Here's how the part is built. I have some questions about the finished solid (model axes, mm). A direction names the side the tool comes from. Round coordinates to 2 decimals unless told otherwise and drop trailing zeros. Order: outer loops, then holes, each group sorted by start corner. A loop starts at its lowest first (then second) coordinate and runs counter-clockwise, first axis right, second up. Notation, with made-up numbers: (1, -9.5) -> (47, -9.5) arc R19 cw to (47, 7.5) -> close; hole circle Ø5 at (-5, 15.5). An arc over 180 degrees is marked (long way). Use a Markdown table: item, result. Add a question column.
from build123d import *

# Parameters (mm, degrees)
F0_W     = 38.1
F0_H     = 31.75
F1_DEPTH = 25.4
F2_W     = 12.7
F2_H     = 19.3866453245
F3_DEPTH = 25.4
F5_DEPTH = 25.4
F7_DEPTH = 25.4


with BuildPart() as f1:
    # F0 (on Right) → F1 (new body)
    with BuildSketch(Plane.YZ):
        with Locations((19.05, 15.875)):
            Rectangle(F0_W, F0_H)
    extrude(amount=F1_DEPTH)

    # F2 (on face) → F3 (cut)
    with BuildSketch(Plane.YZ.offset(25.4)):
        with Locations((6.35, 22.0566773377)):
            Rectangle(F2_W, F2_H)
    extrude(amount=-F3_DEPTH, mode=Mode.SUBTRACT)

    # F4 (on face) → F5 (cut)
    with BuildSketch(Plane(origin=(0, 38.1, 0), x_dir=(-1, 0, 0), z_dir=(0, 1, 0))):
        Polygon((-25.4, 10.1520223543), (-12.7, 31.75), (-25.4, 31.75), align=None)
    extrude(amount=-F5_DEPTH, mode=Mode.SUBTRACT)

    # F6 (on face) → F7 (cut)
    with BuildSketch(Plane.XY.offset(12.3633546755)):
        Polygon((25.4, 0), (25.4, 12.7), (12.7, 0), align=None)
    extrude(amount=-F7_DEPTH, mode=Mode.SUBTRACT)


solid = f1.part
(1) On a 3-axis mill with a long thin cutter (end or side, diameter ignored), from which of +Z, -Z, +X, -X, +Y, -Y can I reach the whole of each face in a straight line? I mean faces 1 (the flat face through (10, 12.7, 22)), 2 (the flat face through (25, 12.7, 12)), 3 (the flat face through (25.4, 25, 5)). Say none if no direction works.
(2) I want a section at C-C on z = 3.5. List the corners of the cut face in (x, y) for me.
(3) I want a section at A-A on y = 32.5. List the corners of the cut face in (x, z) for me.
(4) I want a section at D-D on y = 10. List the corners of the cut face in (x, z) for me, and give its area (3 significant figures).
(5) Please list where these lines run through material, in increasing order: probe 1 along Z at (x, y) = (14.5, 7); probe 2 along Y at (x, z) = (12, 17); probe 3 along Z at (x, y) = (16.75, 21). Write a range as from..to.
(6) I want a section at B-B on x = 9. List the corners of the cut face in (y, z) for me, and give its area (3 significant figures).
(7) I'm going to push flat-ended pins straight in: P1, Ø8, axis at y = 15, z = 24, coming from the +X side; P2, Ø3, axis at x = 15, y = 28.5, coming from the +Z side; P3, Ø12, axis at x = 21.5, z = 14, coming from the -Y side. Where does each tip first touch, or does it pass through?
Output:
| question | item | result |
|---|---|---|
| 1 | face 1 | +Z, +X, -X, -Y |
| 1 | face 2 | +Z, +X, +Y |
| 1 | face 3 | +Z, -Z, +X, +Y, -Y |
| 2 | outline | (0, 0) -> (12.7, 0) -> (25.4, 12.7) -> (25.4, 38.1) -> (0, 38.1) -> close |
| 3 | outline | (0, 0) -> (25.4, 0) -> (25.4, 10.15) -> (12.7, 31.75) -> (0, 31.75) -> close |
| 4 | outline | (0, 0) -> (22.7, 0) -> (22.7, 12.36) -> (0, 12.36) -> close |
| 4 | area | 281 mm² |
| 5 | probe 1 | 0..12.36 |
| 5 | probe 2 | 12.7..38.1 |
| 5 | probe 3 | 0..24.86 |
| 6 | outline | (0, 0) -> (38.1, 0) -> (38.1, 31.75) -> (12.7, 31.75) -> (12.7, 12.36) -> (0, 12.36) -> close |
| 6 | area | 963 mm² |
| 7 | P1 | x = 19.61 |
| 7 | P2 | z = 30.39 |
| 7 | P3 | y = 3.03 |
